Verification items for this drawing (mm, ordinates from the low corner). A direction names the side the tool comes from. Round coordinates to 2 decimals unless told otherwise and drop trailing zeros. Order: outer loops, then holes, each group sorted by start corner. A loop starts at its lowest first (then second) coordinate and runs counter-clockwise, first axis right, second up. Notation, with made-up numbers: (54.5, 45) -> (79.5, 45) arc R19 cw to (79.5, 79) -> close; hole circle Ø1 at (43, -5.5). An arc over 180 degrees is marked (long way). Answer in a Markdown table with one row per item.
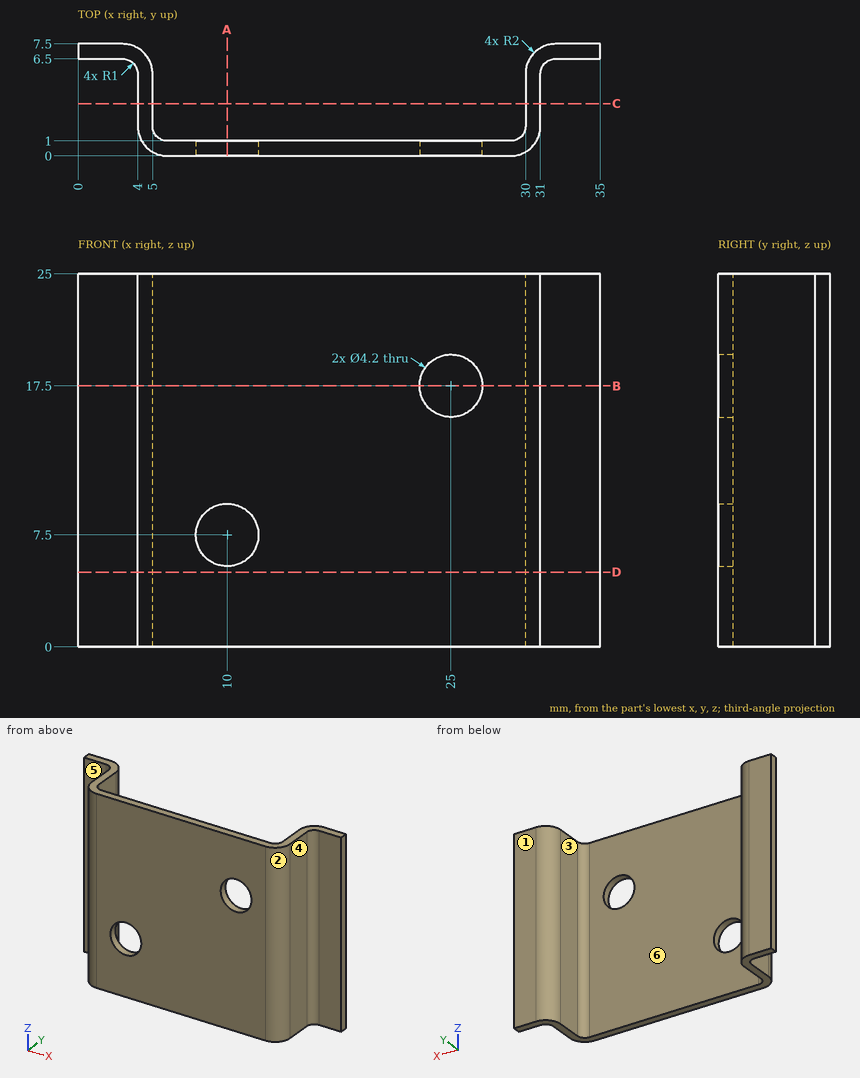
Item 1: Cross-section at C-C (y = 3.5). Record the boundary of the cut face in (x, z), and give its area (3 significant figures).
Result sheet:
| item | result |
|---|---|
| outline | (4, 0) -> (5, 0) -> (5, 25) -> (4, 25) -> close; (30, 0) -> (31, 0) -> (31, 25) -> (30, 25) -> close |
| area | 50.0 mm^2 |
Item 2: Mould release check, pull along X, two halves, no side actions. Record for the marked faces 1, 2 and 3: pulls with the +X half, pulls with the -X half, needs draft (parallel to the pull), parting line crosses it, or undercut.
Result sheet:
| item | result |
|---|---|
| face 1 | needs draft |
| face 2 | pulls with the +X half |
| face 3 | undercut |
Item 3: Scan lines: line 1 (X direction, y = 4.5, z = 13.5); line 2 (Z direction, x = 25, y = 0.75); line 3 (Z direction, x = 10, y = 0.2). Record each from-to range of solid material in increasing order. Write a range as [from, to].
Result sheet:
| item | result |
|---|---|
| line 1 | x = [4, 5], [30, 31] |
| line 2 | z = [0, 15.4], [19.6, 25] |
| line 3 | z = [0, 5.4], [9.6, 25] |
Item 4: Cross-section at B-B (z = 17.5). Record the boundary of the cut face in (x, y).
Result sheet:
| item | result |
|---|---|
| outline | (0, 6.5) -> (3, 6.5) arc R1 cw to (4, 5.5) -> (4, 2) arc R2 ccw to (6, 0) -> (22.9, 0) -> (22.9, 1) -> (6, 1) arc R1 cw to (5, 2) -> (5, 5.5) arc R2 ccw to (3, 7.5) -> (0, 7.5) -> close; (27.1, 0) -> (29, 0) arc R2 ccw to (31, 2) -> (31, 5.5) arc R1 cw to (32, 6.5) -> (35, 6.5) -> (35, 7.5) -> (32, 7.5) arc R2 ccw to (30, 5.5) -> (30, 2) arc R1 cw to (29, 1) -> (27.1, 1) -> close |
Item 5: Depth check by flat-ended pin: P1, Ø1.8, axis at y = 4, z = 14.5, coming from the -X side; P2, Ø6, axis at x = 27.5, z = 19.5, coming from the +Y side; P3, Ø4, axis at y = 3.5, z = 9, coming from the +X side; P4, Ø5.5, axis at x = 10, z = 7.5, coming from the -Y side. Enter the tip coordinate at first touch or a pass-through.
Result sheet:
| item | result |
|---|---|
| P1 | stops at x = 4 |
| P2 | stops at y = 6.82 |
| P3 | stops at x = 31 |
| P4 | stops at y = 0 |
Item 6: Cross-section at D-D (z = 5). Record the boundary of the cut face in (x, y).
Result sheet:
| item | result |
|---|---|
| outline | (0, 6.5) -> (3, 6.5) arc R1 cw to (4, 5.5) -> (4, 2) arc R2 ccw to (6, 0) -> (29, 0) arc R2 ccw to (31, 2) -> (31, 5.5) arc R1 cw to (32, 6.5) -> (35, 6.5) -> (35, 7.5) -> (32, 7.5) arc R2 ccw to (30, 5.5) -> (30, 2) arc R1 cw to (29, 1) -> (6, 1) arc R1 cw to (5, 2) -> (5, 5.5) arc R2 ccw to (3, 7.5) -> (0, 7.5) -> close |
Item 7: Set-up check for the marked faces 4, 5 and 6: record each of +Z, -Z, +X, -X, +Y, -Y from which the full face is reachable in a straight line by a thin tool's end or side.
Result sheet:
| item | result |
|---|---|
| face 4 | +Z, -Z, +X, -Y |
| face 5 | +Z, -Z, -X, -Y |
| face 6 | +Z, -Z, +Y |
Item 8: Cross-section at A-A (x = 10). Record the boundary of the cut face in (y, z), and give its area (3 significant figures).
Result sheet:
| item | result |
|---|---|
| outline | (0, 0) -> (1, 0) -> (1, 5.4) -> (0, 5.4) -> close; (0, 9.6) -> (1, 9.6) -> (1, 25) -> (0, 25) -> close |
| area | 20.8 mm^2 |
